Geometry: final body of the model. Coordinates: model frame, mm. Coordinates: 2 decimals unless noted, no trailing zeros. Write each loop counter-clockwise with the first axis right and the second up, starting at its lowest first coordinate (ties: lowest second). Pieces come first, ordered by that corner, then holes. Notation, with made-up numbers: M 61.25,-0.75 L 76.25,-0.75 A16 cw 76.25,17.25 Z; hole C 20,23.5 d1. An arc over 180 degrees is marked long. Write item = value, one per line. Start each with the question number.
Item 1: Section D-D on z = -1.5. Output: boundary loops of the cut face in (x, y).
Item 2: Ray query, L1, parallel to Y at x = -0.5, z = 4.25; L2, parallel to Z at x = -0.5, y = 1.5. Return the intervals inside material, ascending. Write a range as [from, to].
Item 3: Section A-A on z = 4. Output: boundary loops of the cut face in (x, y).
Item 4: Section C-C on y = 0. Output: boundary loops of the cut face in (x, z), plus the area to 3 significant figures.
Item 5: First-contact query: pin 1 Ø2 at (x, z) = (-1, -1.5) entering from -Y; pin 2 Ø1.5 at (x, y) = (1, 2) entering from -Z. Flat tips, straight axial feed; report the tip coordinate or a pass-through.
Item 6: Section B-B on x = -1.25. Output: boundary loops of the cut face in (y, z).
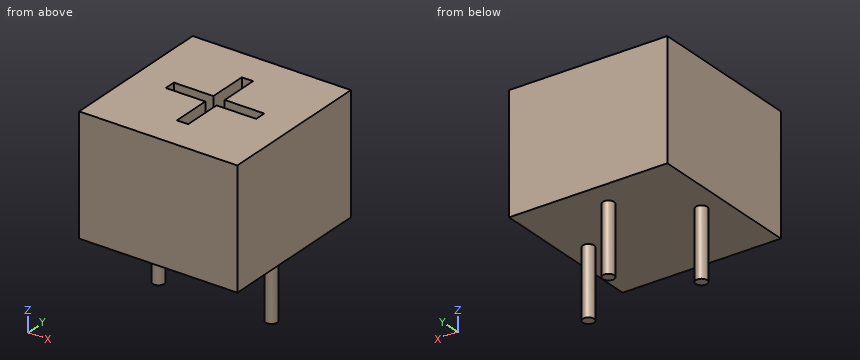
from build123d import *

# Parameters (mm, degrees)
SKETCH1_W           = 7
SKETCH1_H           = 7
BOSS_EXTRUDE1_DEPTH = 5.2
SKETCH2_W           = 4
SKETCH2_H           = 0.5
SKETCH2_W_2         = 0.5
SKETCH2_H_2         = 4
CUT_EXTRUDE1_DEPTH  = 2
SKETCH3_R           = 0.25
BOSS_EXTRUDE2_DEPTH = 3


with BuildPart() as part:
    # Sketch1 → Boss-Extrude1 (new body)
    with BuildSketch(Plane.XY):
        Rectangle(SKETCH1_W, SKETCH1_H)
    extrude(amount=BOSS_EXTRUDE1_DEPTH)

    # Sketch2 → Cut-Extrude1 (cut)
    with BuildSketch(Plane.XY.offset(5.2)):
        Rectangle(SKETCH2_W, SKETCH2_H)
        Rectangle(SKETCH2_W_2, SKETCH2_H_2)
    extrude(amount=-CUT_EXTRUDE1_DEPTH, mode=Mode.SUBTRACT)

    # Sketch3 → Boss-Extrude2 (add)
    with BuildSketch(Plane(origin=(0, 0, 0), x_dir=(-1, 0, 0), z_dir=(0, 0, -1))):
        with Locations((0, 2.25)):
            Circle(SKETCH3_R)
        with Locations((2.5, 0)):
            Circle(SKETCH3_R)
        with Locations((-2.5, 0)):
            Circle(SKETCH3_R)
    extrude(amount=BOSS_EXTRUDE2_DEPTH)


solid = part.part
Responses:
q1.outline = C -2.5,0 d0.5; C 0,2.25 d0.5; C 2.5,0 d0.5
q2.L1 = [-3.5, -0.25], [0.25, 3.5]
q2.L2 = [0, 5.2]
q3.outline = M -3.5,-3.5 L 3.5,-3.5 L 3.5,3.5 L -3.5,3.5 Z; hole M -2,-0.25 L -0.25,-0.25 L -0.25,-2 L 0.25,-2 L 0.25,-0.25 L 2,-0.25 L 2,0.25 L 0.25,0.25 L 0.25,2 L -0.25,2 L -0.25,0.25 L -2,0.25 Z
q4.outline = M -3.5,0 L -2.75,0 L -2.75,-3 L -2.25,-3 L -2.25,0 L 2.25,0 L 2.25,-3 L 2.75,-3 L 2.75,0 L 3.5,0 L 3.5,5.2 L 2,5.2 L 2,3.2 L -2,3.2 L -2,5.2 L -3.5,5.2 Z
q4.area = 31.4 mm²
q5.pin_1 = 2
q5.pin_2 = 0
q6.outline = M -3.5,0 L 3.5,0 L 3.5,5.2 L 0.25,5.2 L 0.25,3.2 L -0.25,3.2 L -0.25,5.2 L -3.5,5.2 Z
